from build123d import *

# Parameters (mm, degrees)
SKETCH_1_R          = 11
EXTRUDE_1_DEPTH     = 5
CHAMFER_1_SIZE      = 3
EXTRUDE_3_DEPTH     = 22
SKETCH_4_W          = 2
SKETCH_4_H          = 7.5
CUT_EXTRUDE_1_DEPTH = 10
SKETCH_6_W          = 2
SKETCH_6_H          = 0.5
EXTRUDE_1_2_DEPTH   = 5
SKETCH_7_W          = 14.2
SKETCH_7_H          = 1.2
EXTRUDE_2_DEPTH     = 1.5


with BuildPart() as part:
    # 草图1 → Extrude 1 (new body)
    with BuildSketch(Plane(origin=(0, 0, 0), x_dir=(1, 0, 0), z_dir=(0, 1, 0))):
        with Locations(Location((0, 0, 0), (0, 0, 270))):
            Circle(SKETCH_1_R)
    extrude(amount=EXTRUDE_1_DEPTH)

    # 倒角1
    chamfer_1_edges = [part.edges().sort_by_distance(p)[0] for p in [
        (0, 0, -11),
    ]]
    chamfer(chamfer_1_edges, length=CHAMFER_1_SIZE)

    # 草图3 → 拉伸3 (add)
    with BuildSketch(Plane(origin=(0, 5, 0), x_dir=(-1, 0, 0), z_dir=(0, 1, 0))):
        with BuildLine():
            Line((-7.9, 5.094114251), (-7.9, -5.094114251))
            ThreePointArc((-7.9, -5.094114251), (0, -9.4), (7.9, -5.094114251))
            Line((7.9, -5.094114251), (7.9, 5.094114251))
            ThreePointArc((7.9, 5.094114251), (0, 9.4), (-7.9, 5.094114251))
        make_face()
    extrude(amount=EXTRUDE_3_DEPTH)

    # 草图4 → 切除-拉伸1 (cut)
    with BuildSketch(Plane(origin=(0, 0, 0), x_dir=(-1, 0, 0), z_dir=(0, 1, 0))):
        Rectangle(SKETCH_4_W, SKETCH_4_H)
    extrude(amount=CUT_EXTRUDE_1_DEPTH, mode=Mode.SUBTRACT)

    # 草图6 → Extrude 1 2 (add)
    with BuildSketch(Plane(origin=(0, 27, 0), x_dir=(1, 0, 0), z_dir=(0, 1, 0))):
        with Locations((4.9, 2.35)):
            Rectangle(SKETCH_6_W, SKETCH_6_H)
        with Locations((-4.9, 2.35)):
            Rectangle(SKETCH_6_W, SKETCH_6_H)
        with Locations((4.9, -2.35)):
            Rectangle(SKETCH_6_W, SKETCH_6_H)
        with Locations((-4.9, -2.35)):
            Rectangle(SKETCH_6_W, SKETCH_6_H)
    extrude(amount=EXTRUDE_1_2_DEPTH)

    # 草图7 → 凸台-拉伸2 (add)
    with BuildSketch(Plane(origin=(0, 27, 0), x_dir=(1, 0, 0), z_dir=(0, 1, 0))):
        Rectangle(SKETCH_7_W, SKETCH_7_H)
    extrude(amount=EXTRUDE_2_DEPTH)


solid = part.part
Verification items for the finished model (mm, model axes). A direction names the side the tool comes from. Coordinates: 2 decimals unless noted, no trailing zeros. Loops run counter-clockwise (first coordinate to the right, second up) from the corner with the lowest first, then second, coordinate; pieces in that order, holes last. Notation, with made-up numbers: (80, -25) -> (86, -25) arc R34 ccw to (86, 8) -> close; hole circle Ø10 at (14.5, -5). An arc over 180 degrees is marked (long way). Answer as a JSON object with one key per item and string values. Group by question number.
Item 1: Mould release check, pull along X, two halves, no side actions. Record for faces 1 (the flat face through (7.1, 28, 0)), 2 (the conical face through (-7.952, 0.146, -1.766)), 3 (the flat face through (5, 29, -2.1)), 4 (the flat face through (-1, 5, 0)): +X half, -X half, draft (parallel to the pull), parting line (faces both ways), or undercut.
Item 2: Sectioned sample at A-A on y = 29. Record the boundary of the cut face in (x, z).
Item 3: Depth check by flat-ended pin: pin 1 (10 mm diameter, centred on x = -5.5, y = 19.5, fed in from -Z); pin 2 (10 mm diameter, centred on y = 10.5, z = 5, fed in from +X); pin 3 (12 mm diameter, centred on x = -1.5, y = 23, fed in from +Z). Enter the tip coordinate at first touch or a pass-through.
Item 4: Tool access check on faces 5 (the flat face through (0, 5, 3.75)), 6 (the cylindrical face through (-0.1, 15.8, 9.4)), 7 (the flat face through (-8.1, 5, 1.6)). Record the directions out of +Z, -Z, +X, -X, +Y, -Y that give a thin tool (end or side, any length) a straight path to the whole face; none if there is none.
Item 5: Scan lines: probe 1 along Z at (x, y) = (-4.5, 28); probe 2 along X at (y, z) = (19.5, -3.25); probe 3 along Y at (x, z) = (-7.25, -0.75). Record each from-to range of solid material in increasing order.
Item 6: Sectioned sample at B-B on z = 0. Record the boundary of the cut face in (x, y).
Item 7: Sectioned sample at D-D on y = 3.5. Record the boundary of the cut face in (x, z), plus the area to 3 significant figures.
Item 8: Sectioned sample at C-C on x = 0. Record the boundary of the cut face in (y, z), plus the area to 3 significant figures.
Evaluation:
{
 "1": {"face 1": "+X half", "face 2": "parting line", "face 3": "draft", "face 4": "undercut"},
 "2": {"outline": "(-5.9, -2.6) -> (-3.9, -2.6) -> (-3.9, -2.1) -> (-5.9, -2.1) -> close; (-5.9, 2.1) -> (-3.9, 2.1) -> (-3.9, 2.6) -> (-5.9, 2.6) -> close; (3.9, -2.6) -> (5.9, -2.6) -> (5.9, -2.1) -> (3.9, -2.1) -> close; (3.9, 2.1) -> (5.9, 2.1) -> (5.9, 2.6) -> (3.9, 2.6) -> close"},
 "3": {"pin 1": "stops at z = -9.39", "pin 2": "stops at x = 7.9", "pin 3": "stops at z = 9.4"},
 "4": {"face 5": "-Y", "face 6": "+Z, +Y", "face 7": "+Y"},
 "5": {"probe 1": "z = -2.6 to -2.1, -0.6 to 0.6, 2.1 to 2.6", "probe 2": "x = -7.9 to 7.9", "probe 3": "y = 0 to 27"},
 "6": {"outline": "(-11, 3) -> (-8, 0) -> (-1, 0) -> (-1, 10) -> (1, 10) -> (1, 0) -> (8, 0) -> (11, 3) -> (11, 5) -> (7.9, 5) -> (7.9, 27) -> (7.1, 27) -> (7.1, 28.5) -> (-7.1, 28.5) -> (-7.1, 27) -> (-7.9, 27) -> (-7.9, 5) -> (-11, 5) -> close"},
 "7": {"outline": "circle Ø22 at (0, 0); hole (-1, -3.75) -> (1, -3.75) -> (1, 3.75) -> (-1, 3.75) -> close", "area": "365 mm²"},
 "8": {"outline": "(0, -8) -> (3, -11) -> (5, -11) -> (5, -9.4) -> (27, -9.4) -> (27, -0.6) -> (28.5, -0.6) -> (28.5, 0.6) -> (27, 0.6) -> (27, 9.4) -> (5, 9.4) -> (5, 11) -> (3, 11) -> (0, 8) -> (0, 3.75) -> (10, 3.75) -> (10, -3.75) -> (0, -3.75) -> close", "area": "441 mm²"}
}
